Study the drawing (mm; zero at the part's minimum x, y, z) and answer. A direction names the side the tool comes from. Round coordinates to 2 decimals unless told otherwise and drop trailing zeros. Loops run counter-clockwise (first coordinate to the right, second up) from the corner with the lowest first, then second, coordinate; pieces in that order, holes last. Notation, with made-up numbers: (72.5, 11.25) - (97.5, 11.25) arc R15 ccw to (97.5, 18.25) - close; hole circle Ø3 at (-12, 33). An arc over 180 degrees is marked (long way). One line per item, written item: value.
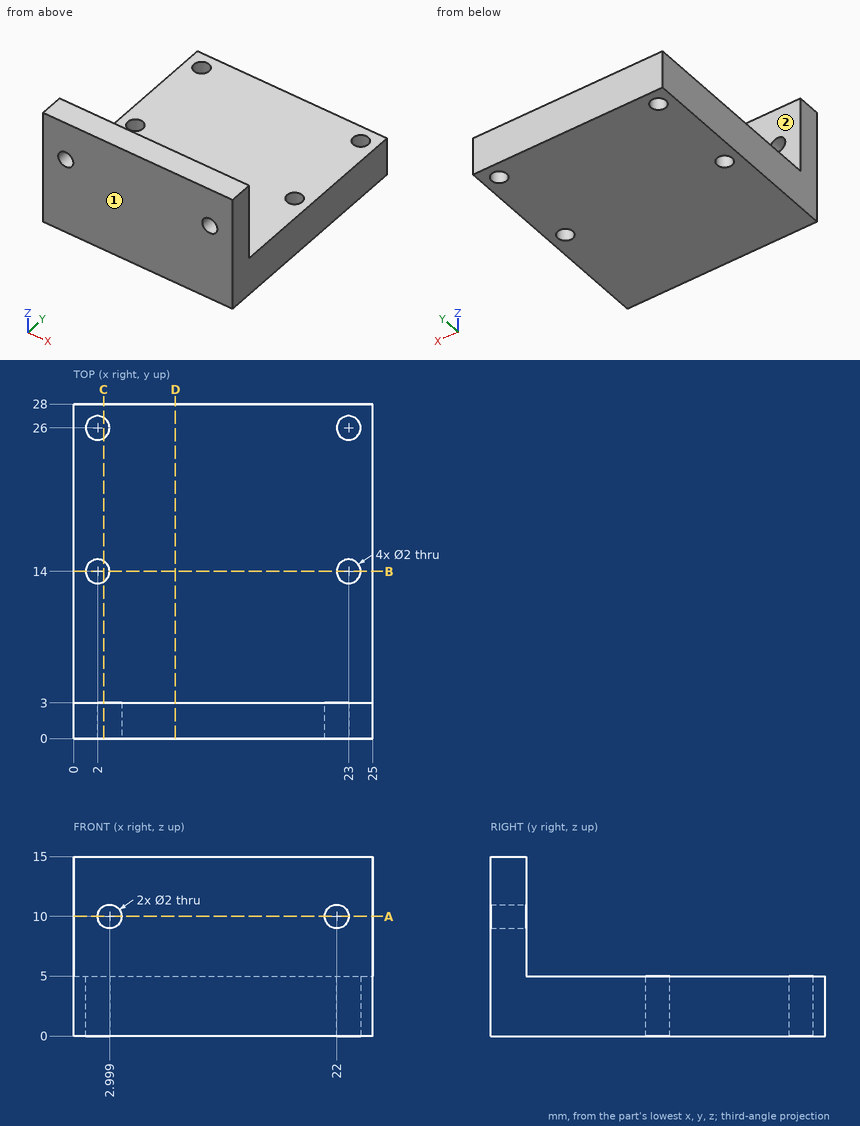
1) Consider L1, parallel to Y at x = 2, z = 1.9; L2, parallel to X at y = 2.35, z = 10; L3, parallel to Z at x = 13.25, y = 26.75. Determine where each line is inside the solid, lowest interval first.
Final values:
L1: 0 to 13, 15 to 25, 27 to 28
L2: 0 to 2, 4 to 21, 23 to 25
L3: 0 to 5
2) For the marked faces 1 and 2, determine the directions among +Z, -Z, +X, -X, +Y, -Y from which every point of the face is accessible in a straight line to the end or side of a thin tool.
Final values:
face 1: +Z, -Z, +X, -X, -Y
face 2: +Z, +X, -X, +Y
3) A cutting plane is placed at C-C on x = 2.5. Give the vertices of the cut face in (y, z).
Final values:
outline: (0, 0) - (13.13, 0) - (13.13, 5) - (3, 5) - (3, 9.13) - (0, 9.13) - close; (0, 10.87) - (3, 10.87) - (3, 15) - (0, 15) - close; (14.87, 0) - (25.13, 0) - (25.13, 5) - (14.87, 5) - close; (26.87, 0) - (28, 0) - (28, 5) - (26.87, 5) - close
4) A cutting plane is placed at A-A on z = 10. Give the vertices of the cut face in (x, y).
Final values:
outline: (0, 0) - (2, 0) - (2, 3) - (0, 3) - close; (4, 0) - (21, 0) - (21, 3) - (4, 3) - close; (23, 0) - (25, 0) - (25, 3) - (23, 3) - close
5) Each of these flat-tipped pins is pushed along its axis until it touches: pin 1 Ø5 at (x, z) = (9, 10.5) entering from +Y; pin 2 Ø1.6 at (x, z) = (3, 10) entering from +Y; pin 3 Ø8 at (x, z) = (9.5, 6.5) entering from +Y; pin 4 Ø3 at (x, y) = (2, 14) entering from +Z. Where does it stop, or does it pass through?
Final values:
pin 1: y = 3
pin 2: through
pin 3: y = 28
pin 4: z = 5
6) A cutting plane is placed at B-B on y = 14. Give the vertices of the cut face in (x, z), and give its area (3 significant figures).
Final values:
outline: (0, 0) - (1, 0) - (1, 5) - (0, 5) - close; (3, 0) - (22, 0) - (22, 5) - (3, 5) - close; (24, 0) - (25, 0) - (25, 5) - (24, 5) - close
area: 105 mm2
7) A cutting plane is placed at D-D on x = 8.5. Give the vertices of the cut face in (y, z), and give its area (3 significant figures).
Final values:
outline: (0, 0) - (28, 0) - (28, 5) - (3, 5) - (3, 15) - (0, 15) - close
area: 170 mm2
